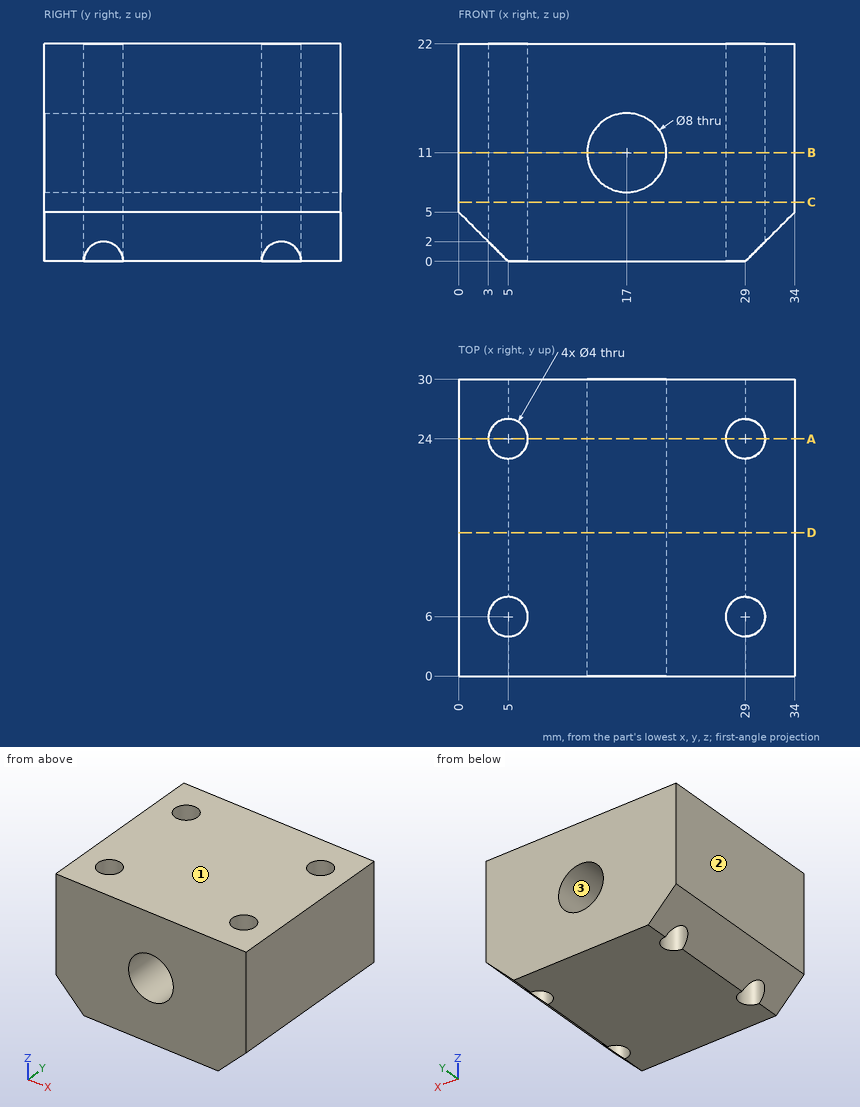
Print and shaded views of the part. All mm, measured from the part's lowest x, y and z. Give positions to 0.01 mm unless a question says otherwise; leave off trailing zeros. Loops run counter-clockwise (first coordinate to the right, second up) from the corner with the lowest first, then second, coordinate; pieces in that order, holes last. Notation, with made-up numbers: (25.25, 67) -> (43.25, 67) arc R13 cw to (43.25, 91) -> close; hole circle Ø2 at (21, 78). An arc over 180 degrees is marked (long way). Use CSV: the item, a comma, the result in double quotes. Start each with the question number.
1) Mould opens along X. For the marked faces 1, 2 and 3 say: released by +X, released by -X, zero draft, split by the parting line, or undercut.
2) Slice it at A-A on y = 24. Give the cut face in (x, z), plus the area to 3 significant figures.
3) Slice it at C-C on z = 6. Give the cut face in (x, y).
4) Wall check: line 1 (Y direction, x = 29, z = 12.5); line 2 (X direction, y = 6.75, z = 8); line 3 (X direction, y = 7.5, z = 18). Give the ranges that are in metal, low to high.
5) Slice it at D-D on y = 14.5. Give the cut face in (x, z).
6) Slice it at B-B on z = 11. Give the cut face in (x, y), plus the area to 3 significant figures.
Computed values:
1,face 1,"zero draft"
1,face 2,"released by -X"
1,face 3,"undercut"
2,outline,"(0, 5) -> (3, 2) -> (3, 22) -> (0, 22) -> close; (7, 0) -> (27, 0) -> (27, 22) -> (7, 22) -> close; (31, 2) -> (34, 5) -> (34, 22) -> (31, 22) -> close; hole circle Ø8 at (17, 11)"
2,area,"501 mm^2"
3,outline,"(0, 0) -> (34, 0) -> (34, 30) -> (0, 30) -> close; hole circle Ø4 at (5, 6); hole circle Ø4 at (5, 24); hole circle Ø4 at (29, 6); hole circle Ø4 at (29, 24)"
4,line 1,"y = 0 to 4, 8 to 22, 26 to 30"
4,line 2,"x = 0 to 3.15, 6.85 to 14.35, 19.65 to 27.15, 30.85 to 34"
4,line 3,"x = 0 to 3.68, 6.32 to 27.68, 30.32 to 34"
5,outline,"(0, 5) -> (5, 0) -> (29, 0) -> (34, 5) -> (34, 22) -> (0, 22) -> close; hole circle Ø8 at (17, 11)"
6,outline,"(0, 0) -> (13, 0) -> (13, 30) -> (0, 30) -> close; (21, 0) -> (34, 0) -> (34, 30) -> (21, 30) -> close; hole circle Ø4 at (5, 6); hole circle Ø4 at (5, 24); hole circle Ø4 at (29, 6); hole circle Ø4 at (29, 24)"
6,area,"730 mm^2"
